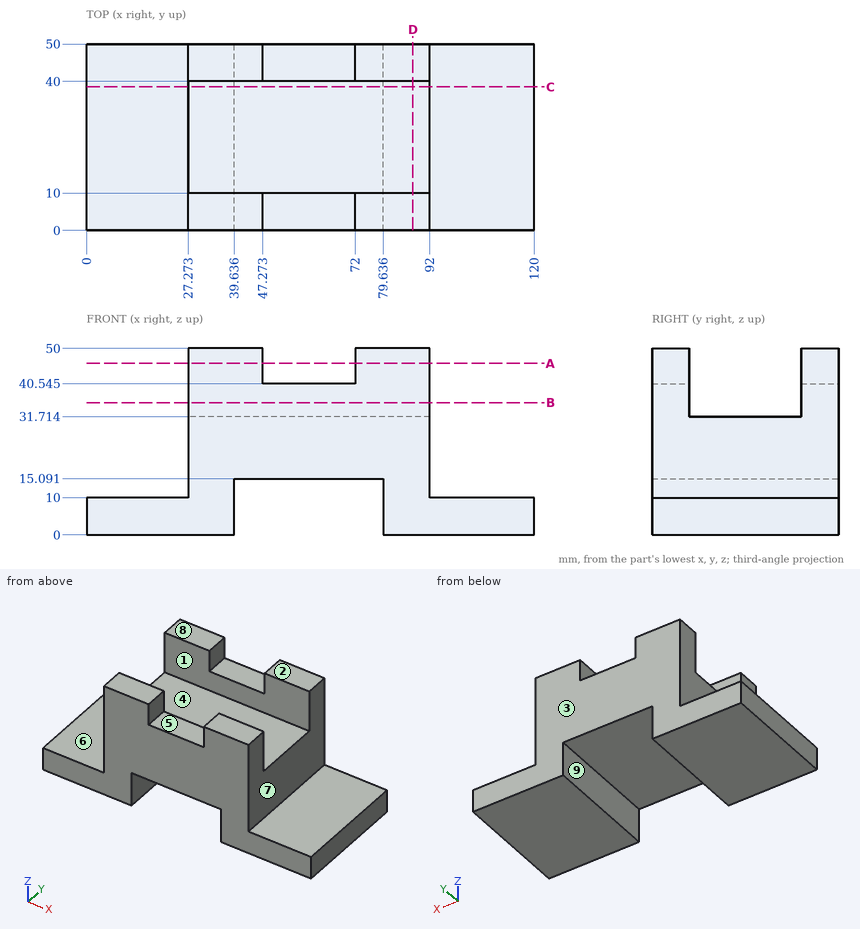
The drawing under review shows one solid part. Ordinate dimensions are in mm from its lowest x, y, z. A direction names the side the tool comes from. Give positions to 0.01 mm unless a question says otherwise; leave off trailing zeros. Order: outer loops, then holes, each group sorted by start corner. A loop starts at its lowest first (then second) coordinate and runs counter-clockwise, first axis right, second up. Notation, with made-up numbers: M 59,62 L 96,62 A36 ccw 96,101 Z; hole C -37.75,1.5 d10. An arc over 180 degrees is marked long. Answer in a Markdown table with one row per item. Add a question column.
1. Add section B-B on z = 35.5. State the section outline as (x, y) points, plus the area to 3 significant figures.
2. Machinability: for the marked faces 5, 6, 7, 8 and 9, which of the approach directions +Z, -Z, +X, -X, +Y, -Y give a long, thin tool a straight path to every point of the face, cutting with its end or side? Answer none if there is none.
3. For pin 1 Ø10.5 at (y, z) = (46, 44.5) entering from +X; pin 2 Ø20 at (x, z) = (57.5, 43) entering from -Y; pin 3 Ø1.5 at (y, z) = (18, 15) entering from -X; pin 4 Ø15 at (x, y) = (49, 19.5) entering from +Z, all flat-tipped, find the tip position at first contact; note any pin that passes through.
4. To check wall thickness, follow line 1 along Y through (x, z) = (54, 32); line 2 along X through (y, z) = (35, 7); line 3 along Z through (x, y) = (14.5, 34). State the ranges of each line that lie inside material, in increasing order.
5. Mouldability with a two-part tool opening along Y and no side actions: class the marked faces 1, 2, 3 and 4 as released by +Y, released by -Y, zero draft, split by the parting line, or undercut.
6. Add section C-C on y = 38.5. State the section outline as (x, z) points.
7. Add section D-D on x = 87.5. State the section outline as (y, z) points, plus the area to 3 significant figures.
8. Add section A-A on z = 46. State the section outline as (x, y) points.
The answers:
| question | item | result |
|---|---|---|
| 1 | outline | M 27.27,0 L 92,0 L 92,10 L 27.27,10 Z; M 27.27,40 L 92,40 L 92,50 L 27.27,50 Z |
| 1 | area | 1,290 mm2 |
| 2 | face 5 | +Z, +Y, -Y |
| 2 | face 6 | +Z, -X, +Y, -Y |
| 2 | face 7 | +Z, +X, +Y, -Y |
| 2 | face 8 | +Z, +X, -X, +Y, -Y |
| 2 | face 9 | -Z, +Y, -Y |
| 3 | pin 1 | x = 92 |
| 3 | pin 2 | y = 0 |
| 3 | pin 3 | x = 27.27 |
| 3 | pin 4 | z = 31.71 |
| 4 | line 1 | 0 to 10, 40 to 50 |
| 4 | line 2 | 0 to 39.64, 79.64 to 120 |
| 4 | line 3 | 0 to 10 |
| 5 | face 1 | undercut |
| 5 | face 2 | zero draft |
| 5 | face 3 | released by +Y |
| 5 | face 4 | undercut |
| 6 | outline | M 0,0 L 39.64,0 L 39.64,15.09 L 79.64,15.09 L 79.64,0 L 120,0 L 120,10 L 92,10 L 92,31.71 L 27.27,31.71 L 27.27,10 L 0,10 Z |
| 7 | outline | M 0,0 L 50,0 L 50,50 L 40,50 L 40,31.71 L 10,31.71 L 10,50 L 0,50 Z |
| 7 | area | 1,950 mm2 |
| 8 | outline | M 27.27,0 L 47.27,0 L 47.27,10 L 27.27,10 Z; M 27.27,40 L 47.27,40 L 47.27,50 L 27.27,50 Z; M 72,0 L 92,0 L 92,10 L 72,10 Z; M 72,40 L 92,40 L 92,50 L 72,50 Z |
